Here's how the part is built. I have some questions about the finished solid (model axes, mm). A direction names the side the tool comes from. Give positions to 0.01 mm unless a question says otherwise; leave off trailing zeros. Loops run counter-clockwise (first coordinate to the right, second up) from the corner with the lowest first, then second, coordinate; pieces in that order, holes last.
Q1. If we section it at A-A (x = 0): Please give me the cut outline in (y, z), plus the area to 3 significant figures.
Q2. We'd pull the mould along X, two halves only. Please class faces 4 (the face through (-2.181, 16.607, -0.255)), 5 (the face through (0, -17, -4)), 6 (the face through (-9.69, 27.31, -0.25)), 7 (the face through (-0.462, -17.544, -8.033)): +X half, -X half, draft (parallel to the pull), parting line (faces both ways), or undercut.
Q3. If we section it at D-D (z = -3): Please give me the cut outline in (x, y), plus the area to 3 significant figures.
Q4. For faces 1 (the face through (14.19, -9.51, -2.8)), 2 (the face through (0, -17, 4)), 3 (the face through (9.883, 26.703, -0.255)), which set-ups out of +Z, -Z, +X, -X, +Y, -Y let a thin tool reach every point of the face, with its end or its side?
Q5. If we section it at B-B (y = 0): Please give me the cut outline in (x, z).
Q6. I need wall thicknesses on line 1 (Y direction, x = 0, z = 5); line 2 (X direction, y = 4.5, z = -2.5); line 3 (X direction, y = 7, z = -0.5). Which ranges of each line are inside material? Lowest first, please.
Q7. Will these pins go through, and if not, where does the flat tip stop? P1, Ø4, axis at x = 2, z = 7.5, coming from the -Y side; P2, Ø4, axis at y = 4.5, z = -8.5, coming from the -X side; P3, Ø2, axis at y = 19.5, z = 5, coming from the -X side; P4, Ø3, axis at y = 19, z = -12.5, coming from the -X side.
Q8. If we section it at C-C (x = -4): Please give me the cut outline in (y, z), plus the area to 3 significant figures.
from build123d import *

# Parameters (mm, degrees)
F0_R          = 16.75
F1_DEPTH      = 17
F1_DEPTH_BACK = 18
F3_DEPTH      = 4
F3_DEPTH_BACK = 4
F4_R          = 3.99999


# Not quite as in the source:
# - a fillet or chamfer is up to 0.001 mm smaller than in the source, because OpenCascade refuses the exact size
# - a feature of the source that left no trace in its solid (it failed there, or was rolled back) is left out


with BuildPart() as f1:
    # F0 (on Top) → F1 (new body, two sides)
    with BuildSketch(Plane.XY) as f1_sk:
        with BuildLine():
            Line((-2.8573335724, 48.6641361257), (-16.7154013983, 5.3476963351))
            ThreePointArc((-16.7154013983, 5.3476963351), (0, -17.55), (16.7154013983, 5.3476963351))
            Line((16.7154013983, 5.3476963351), (2.8573335724, 48.6641361257))
            ThreePointArc((2.8573335724, 48.6641361257), (0, 50.75), (-2.8573335724, 48.6641361257))
        make_face()
        Circle(F0_R, mode=Mode.SUBTRACT)
    extrude(amount=F1_DEPTH)
    extrude(f1_sk.sketch, amount=-F1_DEPTH_BACK)

    # F2 (on Top) → F3 (cut, two sides)
    with BuildSketch(Plane.XY) as f3_sk:
        with BuildLine():
            Line((15.1987458364, -8.775), (0, 0))
            Line((0, 0), (-15.1987458364, -8.775))
            ThreePointArc((-15.1987458364, -8.775), (0, -17.55), (15.1987458364, -8.775))
        make_face()
    extrude(amount=F3_DEPTH, mode=Mode.SUBTRACT)
    extrude(f3_sk.sketch, amount=-F3_DEPTH_BACK, mode=Mode.SUBTRACT)

    # F4 (radius 4 in the source; OpenCascade refuses exactly that, so slightly less here)
    f4_edges = [f1.edges().sort_by_distance(p)[0] for p in [
        (-14.852336, -8.575, 4),
        (-14.852336, -8.575, -4),
        (14.852336, -8.575, -4),
        (14.852336, -8.575, 4),
    ]]
    fillet(f4_edges, radius=F4_R)


solid = f1.part
Check sheet entries:
1. outline: (-17.55, -18) - (-16.75, -18) - (-16.75, -4) - (-17.55, -4) - close; (-17.55, 4) - (-16.75, 4) - (-16.75, 17) - (-17.55, 17) - close; (16.75, -18) - (50.75, -18) - (50.75, 17) - (16.75, 17) - close
1. area: 1,210 mm2
2. face 4: undercut
2. face 5: draft
2. face 6: -X half
2. face 7: parting line
3. outline: (-16.72, 5.35) arc R17.55 ccw to (-14.48, -9.92) - (-13.78, -9.52) arc R16.75 cw (long way) to (13.78, -9.52) - (14.48, -9.92) arc R17.55 ccw to (16.72, 5.35) - (2.86, 48.66) arc R3 ccw to (-2.86, 48.66) - close
3. area: 617 mm2
4. face 1: -Y
4. face 2: +X, -X, -Y
4. face 3: +Z, -Z, +X, +Y
5. outline: (-17.55, -18) - (-16.75, -18) - (-16.75, 17) - (-17.55, 17) - close; (16.75, -18) - (17.55, -18) - (17.55, 17) - (16.75, 17) - close
6. line 1: y = -17.55 to -16.75, 16.75 to 50.75
6. line 2: x = -16.96 to -16.13, 16.13 to 16.96
6. line 3: x = -16.19 to -15.22, 15.22 to 16.19
7. P1: stops at y = -17.55
7. P2: stops at x = -17.37
7. P3: stops at x = -12.51
7. P4: stops at x = -12.83
8. outline: (-17.09, -18) - (-16.27, -18) - (-16.27, -4) - (-17.09, -4) - close; (-17.09, 4) - (-16.27, 4) - (-16.27, 17) - (-17.09, 17) - close; (16.27, -18) - (45.09, -18) - (45.09, 17) - (16.27, 17) - close
8. area: 1,030 mm2
